Geometry check sheet. Reference: the model listing, model coordinates, mm. Coordinates: 2 decimals unless noted, no trailing zeros. Write each loop counter-clockwise with the first axis right and the second up, starting at its lowest first coordinate (ties: lowest second). Pieces come first, ordered by that corner, then holes. Notation, with made-up numbers: (17, -18) -> (38, -18) arc R20 ccw to (38, 12) -> close; hole circle Ø10 at (27.25, -29.5). An arc over 180 degrees is marked (long way). Put each result on its own line as item: value. Start each with the question number.
from build123d import *

# Parameters (mm, degrees)
SKETCH1_W                = 60
SKETCH1_H                = 60
BOSS_EXTRUDE1_DEPTH      = 1
F_4_0_4_DIAMETER_HOLE1_D = 4
ICELL_DEPTH              = 10


with BuildPart() as part:
    # Sketch1 → Boss-Extrude1 (new body)
    with BuildSketch(Plane(origin=(0, 0, 0), x_dir=(1, 0, 0), z_dir=(0, 1, 0))):
        Rectangle(SKETCH1_W, SKETCH1_H)
    extrude(amount=BOSS_EXTRUDE1_DEPTH)

    # Ø4.0 (4) Diameter Hole1 (through all)
    with Locations(Plane(origin=(0, 1, 0), x_dir=(1, 0, 0), z_dir=(0, 1, 0))):
        with Locations((26, 26), (0, 26), (-26, 26), (0, -26), (26, -26), (-26, -26)):
            Hole(F_4_0_4_DIAMETER_HOLE1_D / 2)

    # Sketch19 → iCell (cut)
    with BuildSketch(Plane(origin=(0, 1, 0), x_dir=(1, 0, 0), z_dir=(0, 1, 0))):
        with BuildLine():
            ThreePointArc((-6.5, -0.5), (-7, 0), (-6.5, 0.5))
            add(Edge.make_bspline(
                [(-6.5, 0.5), (-4.333333334, 0.5), (-2.166666667, 4.000004082), (-1e-09, 4.000013237)],
                knots=[0.083333333, 0.083333333, 0.083333333, 0.083333333, 0.916666667, 0.916666667, 0.916666667, 0.916666667], degree=3))
            add(Edge.make_bspline(
                [(6.499999999, 0.5), (4.333333333, 0.5), (2.166666666, 4.000004083), (-1e-09, 4.000013237)],
                knots=[0.083333333, 0.083333333, 0.083333333, 0.083333333, 0.916666667, 0.916666667, 0.916666667, 0.916666667], degree=3))
            ThreePointArc((6.499999999, 0.5), (6.999999999, 0), (6.499999999, -0.5))
            add(Edge.make_bspline(
                [(6.499999999, -0.5), (4.333333333, -0.5), (2.166666666, -4.000004083), (0, -4.000013237)],
                knots=[0.083333333, 0.083333333, 0.083333333, 0.083333333, 0.916666667, 0.916666667, 0.916666667, 0.916666667], degree=3))
            add(Edge.make_bspline(
                [(-6.5, -0.5), (-4.333333334, -0.5), (-2.166666667, -4.000004083), (0, -4.000013237)],
                knots=[0.083333333, 0.083333333, 0.083333333, 0.083333333, 0.916666667, 0.916666667, 0.916666667, 0.916666667], degree=3))
        make_face()
    extrude(amount=-ICELL_DEPTH, mode=Mode.SUBTRACT)


solid = part.part
Item 1: Section check B-B, the plane z = -26. Enter the section's corners in (x, y), and give its area (3 significant figures).
Item 2: Section check A-A, the plane x = -26. Enter the section's corners in (y, z).
Item 3: Mould release check, pull along Z, two halves, no side actions. Record for faces 1 (the cylindrical face through (-25.566, 0.493, -24.048)), 2 (the flat face through (-7.1, 0, -0.4)), 3 (the cylindrical face through (0.434, 0.493, 27.952)): released by +Z, released by -Z, zero draft, split by the parting line, or undercut.
Item 4: Scan lines: line 1 along X through (y, z) = (0.7, 26); line 2 along Z through (x, y) = (-26, 0.2); line 3 along Z through (x, y) = (0, 0.35). Record each from-to range of solid material in increasing order. Write a range as [from, to].
Item 5: Go/stop test with a flat-tipped pin: P1, Ø3, axis at x = 26, z = 26, coming from the -Y side. Record where the tip stops, or that it passes through.
Item 6: Section check C-C, the plane y = 0.2. Give the number of separate pieces and of enclosed holes in the cut face, and give its area (3 significant figures).
From the geometry:
1. outline: (-30, 0) -> (-28, 0) -> (-28, 1) -> (-30, 1) -> close; (-24, 0) -> (-2, 0) -> (-2, 1) -> (-24, 1) -> close; (2, 0) -> (24, 0) -> (24, 1) -> (2, 1) -> close; (28, 0) -> (30, 0) -> (30, 1) -> (28, 1) -> close
1. area: 48.0 mm²
2. outline: (0, -30) -> (1, -30) -> (1, -28) -> (0, -28) -> close; (0, -24) -> (1, -24) -> (1, 24) -> (0, 24) -> close; (0, 28) -> (1, 28) -> (1, 30) -> (0, 30) -> close
3. face 1: undercut
3. face 2: zero draft
3. face 3: undercut
4. line 1: [-30, -28], [-24, -2], [2, 24], [28, 30]
4. line 2: [-30, -28], [-24, 24], [28, 30]
4. line 3: [-30, -28], [-24, -4], [4, 24], [28, 30]
5. P1: through
6. separate pieces: 1
6. enclosed holes: 7
6. area: 3,470 mm²
